Read the model definition and answer for the solid it produces. Units are mm, in the model's axes. Round coordinates to 2 decimals unless told otherwise and drop trailing zeros. Write each loop counter-clockwise with the first axis right and the second up, starting at its lowest first coordinate (ties: lowest second). Pieces come first, ordered by that corner, then holes. Notation, with made-up numbers: M -38,-17.75 L -3,-17.75 A10 cw -3,-11.75 Z; hole C -2,-1 d3. An arc over 180 degrees is marked long. Use one line per item in the form item = value. Start each with the question number.
```python
from build123d import *

# Parameters (mm, degrees)
BOSS_EXTRUDE1_DEPTH = 3.175
SKETCH2_W           = 38.735
SKETCH2_H           = 254
BOSS_EXTRUDE2_DEPTH = 3.175


with BuildPart() as part:
    # Sketch1 → Boss-Extrude1 (new body)
    with BuildSketch(Plane.XY):
        Polygon((0, 0), (0, 381), (152.4, 54.177145314), (152.4, -22.022854686), align=None)
    extrude(amount=BOSS_EXTRUDE1_DEPTH)

    # Sketch2 → Boss-Extrude2 (add)
    with BuildSketch(Plane.XY.offset(3.175)):
        with Locations((-19.3675, 165.1)):
            Rectangle(SKETCH2_W, SKETCH2_H)
    extrude(amount=-BOSS_EXTRUDE2_DEPTH)


solid = part.part
```
Q1. Each of these flat-tipped pins is pushed along its axis until it touches: pin 1 Ø1.6 at (x, z) = (-26.5, 1) entering from +Y; pin 2 Ø1 at (x, z) = (80.5, 1.5) entering from -Y; pin 3 Ø1 at (y, z) = (337.5, 1) entering from -X. Where does it stop, or does it pass through?
Q2. Find section B-B on x = -23. Write down the section's boundary in (y, z) (3 decimals).
Q3. Straight lines are drawn through the part: line 1 (Y direction, x = -29, z = 3.05); line 2 (Y direction, x = 28.5, z = 2.4); line 3 (X direction, y = 212.5, z = 0.4) (3 decimals). For each, find the intervals that lie inside material, in ascending order. Write a range as [from, to].
Q4. Find section A-A on z = 2.55. Write down the section's boundary in (x, y) (3 decimals), and give its area (3 significant figures).
Q5. Find section C-C on y = 7. Write down the section's boundary in (x, z) (3 decimals).
Response:
q1.pin_1 = 292.1
q1.pin_2 = -11.71
q1.pin_3 = 0
q2.outline = M 38.1,0 L 292.1,0 L 292.1,3.175 L 38.1,3.175 Z
q3.line_1 = [38.1, 292.1]
q3.line_2 = [-4.12, 319.88]
q3.line_3 = [-38.735, 78.573]
q4.outline = M -38.735,38.1 L 0,38.1 L 0,0 L 152.4,-22.023 L 152.4,54.177 L 0,381 L 0,292.1 L -38.735,292.1 Z
q4.area = 44,700 mm²
q5.outline = M 0,0 L 152.4,0 L 152.4,3.175 L 0,3.175 Z
